Verification items for the finished model (mm, model axes). A direction names the side the tool comes from. Coordinates: 2 decimals unless noted, no trailing zeros. Order: outer loops, then holes, each group sorted by start corner. A loop starts at its lowest first (then second) coordinate and runs counter-clockwise, first axis right, second up. Notation, with made-up numbers: M 23.25,23 L 42.25,23 A27 cw 42.25,53 Z; hole C -38.75,62.5 d6. An arc over 180 degrees is marked long. Write item = value, one per line.
```python
from build123d import *

# Parameters (mm, degrees)
PAD081_DEPTH          = 12
SKETCH230_R           = 7.15
POCKET159_DEPTH       = 20
POLARPATTERN_COUNT    = 4
PAD106_DEPTH          = 12
PAD105_DEPTH          = 5
SKETCH266_R           = 1.5
POCKET160_DEPTH       = 30
FILLET005_R           = 12
POLARPATTERN002_COUNT = 4
POCKET162_DEPTH       = 5
POCKET178_DEPTH       = 13
CHAMFER044_SIZE       = 0.5


with BuildPart() as part:
    # Sketch232 → Pad081 (new body)
    with BuildSketch(Plane.XY.offset(-10)):
        Polygon((0, 0), (0, 25), (8.9644660941, 16.0355339059), (5.4289321881, 12.5), (8.2573593129, 9.6715728753), (6.8431457505, 8.2573593129), (8.2573593129, 6.8431457505), (9.6715728753, 8.2573593129), (12.5, 5.4289321881), (16.0355339059, 8.9644660941), (25, 0), align=None)
    pad081 = extrude(amount=-PAD081_DEPTH)

    # Sketch230 → Pocket159 (cut)
    with BuildSketch(Plane.XY.offset(-23)):
        Circle(SKETCH230_R)
    pocket159 = extrude(amount=POCKET159_DEPTH, mode=Mode.SUBTRACT)

    # PolarPattern: Pad081, Pocket159 ×4 about axis
    polarpattern_axis = Axis((0, 0, -10), (0, 0, 1))
    for i in range(1, POLARPATTERN_COUNT):
        add(pad081.rotate(polarpattern_axis, i * 360 / POLARPATTERN_COUNT))
        add(pocket159.rotate(polarpattern_axis, i * 360 / POLARPATTERN_COUNT), mode=Mode.SUBTRACT)

    # Sketch297 → Pad106 (join)
    with BuildSketch(Plane.XY.offset(-22)):
        Polygon((-11.965, -19.035), (-5.43, -12.5), (5.43, -12.5), (11.965, -19.035), (6, -25), (-6, -25), align=None)
    extrude(amount=PAD106_DEPTH)

    # Sketch296 → Pad105 (join)
    with BuildSketch(Plane.XZ.offset(25)):
        with BuildLine():
            Line((-3.9127822424, 0.8307437172), (-6, -9))
            Line((-6, -22), (-6, -9))
            Line((6, -22), (-6, -22))
            Line((6, -9), (6, -22))
            Line((3.9127822424, 0.8307437172), (6, -9))
            ThreePointArc((3.9127822424, 0.8307437172), (0, 4), (-3.9127822424, 0.8307437172))
        make_face()
        Polygon((-2.1213203436, 0), (0, -2.1213203436), (2.1213203436, 0), (0, 2.1213203436), align=None, mode=Mode.SUBTRACT)
    extrude(amount=PAD105_DEPTH)

    # Sketch266 (on DatumPlane) → Pocket160 (cut, symmetric)
    with BuildSketch(Plane(origin=(2.8284271247, -2.8284271247, 0), x_dir=(0.7071067812, 0.7071067812, 0), z_dir=(0.7002252666, -0.7002252666, -0.139173101))):
        with Locations((14, -16.5)):
            Circle(SKETCH266_R)
    pocket160 = extrude(amount=POCKET160_DEPTH, both=True, mode=Mode.SUBTRACT)

    # Fillet005
    fillet005_edges = [part.edges().sort_by_distance(p)[0] for p in [
        (-6, -25, -16),
        (6, -25, -16),
    ]]
    fillet(fillet005_edges, radius=FILLET005_R)

    # PolarPattern002: Pocket160 ×4 about axis
    polarpattern002_axis = Axis((0, 0, 0), (0, 0, 1))
    for i in range(1, POLARPATTERN002_COUNT):
        add(pocket160.rotate(polarpattern002_axis, i * 360 / POLARPATTERN002_COUNT), mode=Mode.SUBTRACT)

    # Sketch272 → Pocket162 (cut, symmetric)
    with BuildSketch(Plane.YZ):
        Polygon((20.3, -23), (26, -16.3), (26, -23), align=None)
    extrude(amount=POCKET162_DEPTH, both=True, mode=Mode.SUBTRACT)

    # Sketch303 → Pocket178 (cut)
    with BuildSketch(Plane.XY.offset(-10)):
        Polygon((-5.5, -12.5), (-12, -19), (-10.9393398282, -20.0606601718), align=None)
        Polygon((5.5, -12.5), (12, -19), (10.9393398282, -20.0606601718), align=None)
    extrude(amount=-POCKET178_DEPTH, mode=Mode.SUBTRACT)

    # Chamfer044
    chamfer044_edges = [part.edges().sort_by_distance(p)[0] for p in [
        (-5.055813, 5.055813, -22),
    ]]
    chamfer(chamfer044_edges, length=CHAMFER044_SIZE)


solid = part.part
```
Item 1: Gauge pin test, flat ends, axial feed: pin 1 (3.5 mm diameter, centred on x = 1.5, z = -4, fed in from +Y); pin 2 (3 mm diameter, centred on x = -19.5, y = -2, fed in from +Z); pin 3 (5.5 mm diameter, centred on y = -27, z = -15.5, fed in from -X); pin 4 (5 mm diameter, centred on y = -21, z = -3, fed in from -X). Record the tip position at first contact, or that the pin passes through.
Report:
pin_1 = -25
pin_2 = -10
pin_3 = -7.45
pin_4 = through
Item 2: Sectioned sample at A-A, the plane z = -8.25. Enter the section's corners in (x, y), then the cut area to 3 significant figures.
Report:
outline = M -5.84,-30 L 5.84,-30 L 5.84,-25 L -5.84,-25 Z
area = 58.4 mm^2
Item 3: Tool access check on faces 4 (the flat face through (7.6, -7.5, -15.9)), 5 (the flat face through (14.636, 7.565, -15.916)), 6 (the flat face through (6.82, 11.11, -19.01)). Record the directions out of +Z, -Z, +X, -X, +Y, -Y that give a thin tool (end or side, any length) a straight path to the whole face; none if there is none.
Report:
face_4 = +Z, -Z
face_5 = +Z, -Z, +Y
face_6 = +Z, -Z, +X
Item 4: Scan lines: L1, parallel to Z at x = -0.5, y = 19; L2, parallel to X at y = 14.5, z = -16; L3, parallel to X at y = -20, z = -15. Record each from-to range of solid material in increasing order. Write a range as from..to.
Report:
L1 = -22..-19.44, -16.44..-15.36, -12.96..-10
L2 = -7.43..-7.07, -3.92..3.68, 7.23..7.43
L3 = -10.9..-1.66, 1.72..10.9
Item 5: Release check for a two-part mould opening along Y. For faces 1 (the flat face through (0, -30, -12)), 2 (the flat face through (-7.56, -8.974, -15.916)), 3 (the flat face through (-1.046, -27.465, 1.076)) record: pulls with the +Y half, pulls with the -Y half, needs draft (parallel to the pull), parting line crosses it, or undercut.
Report:
face_1 = pulls with the -Y half
face_2 = undercut
face_3 = needs draft
